Verification items for the finished model (mm, model axes). Face numbers are marked on the shaded views. A direction names the side the tool comes from. Round coordinates to 2 decimals unless told otherwise and drop trailing zeros. Loops run counter-clockwise (first coordinate to the right, second up) from the corner with the lowest first, then second, coordinate; pieces in that order, holes last. Notation, with made-up numbers: (16.5, 62.25) -> (35.5, 62.25) arc R27 cw to (35.5, 98.25) -> close; hole circle Ø5 at (55.5, 87). An arc over 180 degrees is marked (long way). Write item = value, one per line.
```python
from build123d import *

# Parameters (mm, degrees)
SKETCH_1_R          = 50
SKETCH_1_R_2        = 42
SKETCH_1_R_3        = 1.55
EXTRUDE_1_DEPTH     = 10
EXTRUDE_START       = -10
SKETCH_3_R          = 42
SKETCH_3_R_2        = 27.55
EXTRUDE_2_DEPTH     = 10
SKETCH_5_R          = 28.648994564
SKETCH_5_R_2        = 24
EXTRUDE_4_DEPTH     = 3.95
CUT_EXTRUDE_1_DEPTH = 10


with BuildPart() as part:
    # 草图1 → 凸台-拉伸1 (new body)
    with BuildSketch(Plane.XY):
        Circle(SKETCH_1_R)
        Circle(SKETCH_1_R_2, mode=Mode.SUBTRACT)
        with Locations((46, 0)):
            Circle(SKETCH_1_R_3, mode=Mode.SUBTRACT)
        with Locations((23, -39.837168574)):
            Circle(SKETCH_1_R_3, mode=Mode.SUBTRACT)
        with Locations((-23, -39.837168574)):
            Circle(SKETCH_1_R_3, mode=Mode.SUBTRACT)
        with Locations((-46, 0)):
            Circle(SKETCH_1_R_3, mode=Mode.SUBTRACT)
        with Locations((-23, 39.837168574)):
            Circle(SKETCH_1_R_3, mode=Mode.SUBTRACT)
        with Locations((23, 39.837168574)):
            Circle(SKETCH_1_R_3, mode=Mode.SUBTRACT)
    extrude(amount=EXTRUDE_1_DEPTH)

    # 草图3 → 凸台-拉伸2 (add)
    with BuildSketch(Plane.XY.offset(10).offset(EXTRUDE_START)):
        Circle(SKETCH_3_R)
        Circle(SKETCH_3_R_2, mode=Mode.SUBTRACT)
    extrude(amount=EXTRUDE_2_DEPTH)

    # 草图5 → 凸台-拉伸4 (add)
    with BuildSketch(Plane.XY.offset(10)):
        Circle(SKETCH_5_R)
        Circle(SKETCH_5_R_2, mode=Mode.SUBTRACT)
    extrude(amount=-EXTRUDE_4_DEPTH)

    # 草图6 → 切除-拉伸1 (cut)
    with BuildSketch(Plane(origin=(0, 0, 0), x_dir=(-1, 0, 0), z_dir=(0, 0, -1))):
        with BuildLine():
            ThreePointArc((10.083378512, 38.891869692), (-20.088877833, 34.794957074), (-38.72303641, 10.713472899))
            ThreePointArc((-38.72303641, 10.713472899), (-35.810551361, 5.572975291), (-30.670053754, 8.48546034))
            ThreePointArc((-30.670053754, 8.48546034), (-15.911122167, 27.558871999), (7.98640266, 30.803775856))
            ThreePointArc((7.98640266, 30.803775856), (13.078937504, 33.799334848), (10.083378512, 38.891869692))
        make_face()
        with BuildLine():
            ThreePointArc((28.639657898, -28.178396793), (40.177755666, 0), (28.639657898, 28.178396793))
            ThreePointArc((28.639657898, 28.178396793), (22.731613858, 28.226359557), (22.683651094, 22.318315516))
            ThreePointArc((22.683651094, 22.318315516), (31.822244334, 0), (22.683651094, -22.318315516))
            ThreePointArc((22.683651094, -22.318315516), (22.731613858, -28.226359557), (28.639657898, -28.178396793))
        make_face()
        with BuildLine():
            ThreePointArc((-38.72303641, -10.713472899), (-20.088877833, -34.794957074), (10.083378512, -38.891869692))
            ThreePointArc((10.083378512, -38.891869692), (13.078937504, -33.799334848), (7.98640266, -30.803775856))
            ThreePointArc((7.98640266, -30.803775856), (-15.911122167, -27.558871999), (-30.670053754, -8.48546034))
            ThreePointArc((-30.670053754, -8.48546034), (-35.810551361, -5.572975291), (-38.72303641, -10.713472899))
        make_face()
    extrude(amount=-CUT_EXTRUDE_1_DEPTH, mode=Mode.SUBTRACT)


solid = part.part
```
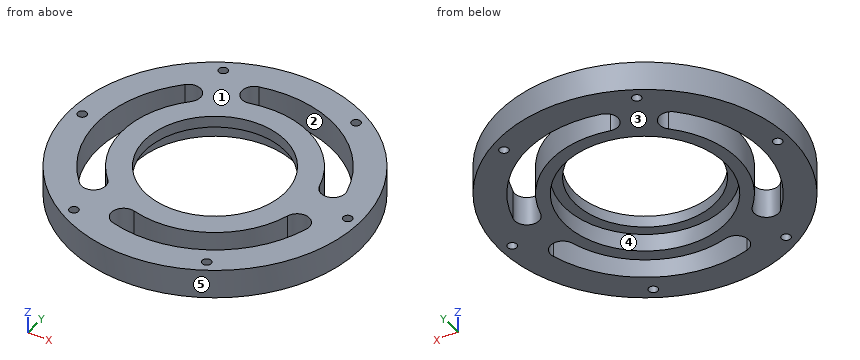
(1) Go/stop test with flat-tipped pins: pin 1 Ø1 at (y, z) = (-35, 1) entering from +X; pin 2 Ø3 at (x, z) = (33, 7.5) entering from -Y; pin 3 Ø5 at (x, z) = (-24, 8.5) entering from -Y. Record where each tip stops, or that it passes through.
Filled sheet:
pin_1 = 36.19
pin_2 = -38.83
pin_3 = -45.14
(2) Material ranges on probe 1 along Y at (x, z) = (-12.5, 5); probe 2 along X at (y, z) = (-28.5, 2.5); probe 3 along X at (y, z) = (-2, 7.75), recorded low to high. Write a range as from..to.
Filled sheet:
probe_1 = -48.41..-37.18, -32.51..-24.55, 24.55..32.51, 37.18..48.41
probe_2 = -41.08..-28.28, -23.04..14.16, 28.32..41.08
probe_3 = -49.96..-40.13, -31.76..-23.92, 23.92..49.96
(3) Sectioned sample at C-C, the plane x = 46. Record the cut outline in (y, z).
Filled sheet:
outline = (-19.6, 0) -> (-1.55, 0) -> (-1.55, 10) -> (-19.6, 10) -> close; (1.55, 0) -> (19.6, 0) -> (19.6, 10) -> (1.55, 10) -> close
(4) Draft check along X on the marked faces 3, 4 and 5. Enter one of: released by +X, released by -X, zero draft, split by the parting line, or undercut.
Filled sheet:
face_3 = zero draft
face_4 = undercut
face_5 = split by the parting line
(5) Set-up check for the marked faces 1 and 2: record each of +Z, -Z, +X, -X, +Y, -Y from which the full face is reachable in a straight line by a thin tool's end or side.
Filled sheet:
face_1 = +Z, +X, -X, +Y, -Y
face_2 = +Z, -Z
(6) Sectioned sample at B-B, the plane x = 0. Record the cut outline in (y, z), and give its area (3 significant figures).
Filled sheet:
outline = (-50, 0) -> (-40.18, 0) -> (-40.18, 10) -> (-50, 10) -> close; (-31.82, 0) -> (-27.55, 0) -> (-27.55, 6.05) -> (-24, 6.05) -> (-24, 10) -> (-31.82, 10) -> close; (24, 6.05) -> (27.55, 6.05) -> (27.55, 0) -> (31.82, 0) -> (31.82, 10) -> (24, 10) -> close; (40.18, 0) -> (50, 0) -> (50, 10) -> (40.18, 10) -> close
area = 310 mm2
(7) Sectioned sample at D-D, the plane y = 17. Record the cut outline in (x, z), and give its area (3 significant figures).
Filled sheet:
outline = (-47.02, 0) -> (-36.4, 0) -> (-36.4, 10) -> (-47.02, 10) -> close; (-26.9, 0) -> (-21.68, 0) -> (-21.68, 6.05) -> (-16.94, 6.05) -> (-16.94, 10) -> (-26.9, 10) -> close; (16.94, 6.05) -> (21.68, 6.05) -> (21.68, 0) -> (26.9, 0) -> (26.9, 10) -> (16.94, 10) -> close; (36.4, 0) -> (47.02, 0) -> (47.02, 10) -> (36.4, 10) -> close
area = 354 mm2
(8) Sectioned sample at A-A, the plane y = 0. Record the cut outline in (x, z).
Filled sheet:
outline = (-50, 0) -> (-47.55, 0) -> (-47.55, 10) -> (-50, 10) -> close; (-44.45, 0) -> (-40.18, 0) -> (-40.18, 10) -> (-44.45, 10) -> close; (-31.82, 0) -> (-27.55, 0) -> (-27.55, 6.05) -> (-24, 6.05) -> (-24, 10) -> (-31.82, 10) -> close; (24, 6.05) -> (27.55, 6.05) -> (27.55, 0) -> (44.45, 0) -> (44.45, 10) -> (24, 10) -> close; (47.55, 0) -> (50, 0) -> (50, 10) -> (47.55, 10) -> close
